```python
from build123d import *

# Parameters (mm, degrees)
SKETCH1_R           = 15.375
SKETCH1_R_2         = 10.375
BOSS_EXTRUDE1_DEPTH = 25
BOSS_EXTRUDE2_START = 52.5
SKETCH3_R           = 15.375
BOSS_EXTRUDE2_DEPTH = 52.5
FILLET1_R           = 2


with BuildPart() as part:
    # Sketch1 → Boss-Extrude1 (new body)
    with BuildSketch(Plane(origin=(0, 0, 0), x_dir=(1, 0, 0), z_dir=(0, 1, 0))):
        with Locations(Location((0, 0, 0), (0, 0, 270))):
            Circle(SKETCH1_R)
        with Locations(Location((0, 0, 0), (0, 0, 270))):
            Circle(SKETCH1_R_2, mode=Mode.SUBTRACT)
    extrude(amount=BOSS_EXTRUDE1_DEPTH)

    # Sketch3 → Boss-Extrude2 (add)
    with BuildSketch(Plane.XZ.offset(BOSS_EXTRUDE2_START)):
        with Locations(Location((0, 0, 0), (0, 0, 270))):
            Circle(SKETCH3_R)
    extrude(amount=-BOSS_EXTRUDE2_DEPTH)

    # Fillet1
    fillet1_edges = [part.edges().sort_by_distance(p)[0] for p in [
        (0, 25, -15.375),
        (0, 0, -10.375),
    ]]
    fillet(fillet1_edges, radius=FILLET1_R)


solid = part.part
```
Read the model definition and answer for the solid it produces. Units are mm, in the model's axes. A direction names the side the tool comes from. Coordinates: 2 decimals unless noted, no trailing zeros. Write each loop counter-clockwise with the first axis right and the second up, starting at its lowest first coordinate (ties: lowest second). Pieces come first, ordered by that corner, then holes. Notation, with made-up numbers: (67.25, 67) - (126.25, 67) arc R11 ccw to (126.25, 80) - close; hole circle Ø6 at (18, 44.25). An arc over 180 degrees is marked (long way). Answer as a JSON object with one key per item and string values. Group by question number.
1. A cutting plane is placed at B-B (z = 0). Determine the outline of the cut face in (x, y) (3 decimals).
2. Consider L1, parallel to X at y = 11.5, z = 0 (3 decimals); L2, parallel to Z at x = 2, y = 2; L3, parallel to Y at x = 3.5, z = 0.5. Determine where each line is inside the solid, lowest interval first. Write a range as [from, to].
3. Each of these flat-tipped pins is pushed along its axis until it touches: P1, Ø13.5, axis at x = -2, z = 0.5, coming from the +Y side; P2, Ø10, axis at x = -1.5, y = -1.5, coming from the -Z side (3 decimals); P3, Ø1, axis at y = -31, z = -1.5, coming from the -X side; P4, Ø1.5, axis at x = -11, y = 14, coming from the -Z side. Where does it stop, or does it pass through?
4. A cutting plane is placed at A-A (x = 0). Determine the outline of the cut face in (y, z) (3 decimals).
5. Which of the six approach directions +Z, -Z, +X, -X, +Y, -Y give full straight-line access (tool end or side, diameter ignored) to faces 1 (the flat face through (0, 0, 0)), 2 (the flat face through (0, -52.5, 0))?
6. A cutting plane is placed at C-C (y = -22). Determine the outline of the cut face in (x, z) (3 decimals).
Worked out:
{
 "1": {"outline": "(-15.375, -52.5) - (15.375, -52.5) - (15.375, 23) arc R2 ccw to (13.375, 25) - (10.375, 25) - (10.375, 2) arc R2 cw to (8.375, 0) - (-8.375, 0) arc R2 cw to (-10.375, 2) - (-10.375, 25) - (-13.375, 25) arc R2 ccw to (-15.375, 23) - close"},
 "2": {"L1": "x = [-15.375, -10.375], [10.375, 15.375]", "L2": "z = [-15.24, -10.18], [10.18, 15.24]", "L3": "y = [-52.5, 0]"},
 "3": {"P1": "stops at y = 0.05", "P2": "stops at z = -15.375", "P3": "stops at x = -15.34", "P4": "stops at z = -11.46"},
 "4": {"outline": "(-52.5, -15.375) - (23, -15.375) arc R2 ccw to (25, -13.375) - (25, -10.375) - (2, -10.375) arc R2 cw to (0, -8.375) - (0, 8.375) arc R2 cw to (2, 10.375) - (25, 10.375) - (25, 13.375) arc R2 ccw to (23, 15.375) - (-52.5, 15.375) - close"},
 "5": {"face 1": "+Y", "face 2": "+Z, -Z, +X, -X, -Y"},
 "6": {"outline": "circle Ø30.75 at (0, 0)"}
}
